Geometry: final body of the model. Coordinates: model frame, mm. Face numbers are marked on the shaded views. Round coordinates to 2 decimals unless told otherwise and drop trailing zeros. Loops run counter-clockwise (first coordinate to the right, second up) from the corner with the lowest first, then second, coordinate; pieces in that order, holes last. Notation, with made-up numbers: (-7, 35) - (-2, 35) arc R28 ccw to (-2, 53) - close; hole circle Ø10 at (-36, -20). An arc over 180 degrees is marked (long way). Answer in a Markdown table with one row per item. Add a question column.
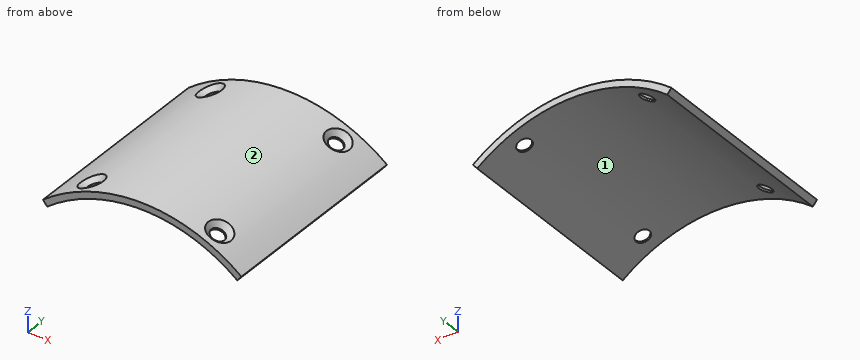
from build123d import *

# Parameters (mm, degrees)
SKETCH1_R           = 76.2
SKETCH1_R_2         = 74.549
BOSS_EXTRUDE1_DEPTH = 254
WRAP2_SECTION_W     = 3.302
WRAP2_SECTION_H     = 101.6
WRAP2_ANGLE         = 76.394372684
SKETCH4_W           = 76.2
SKETCH4_H           = 254


# Read off the part's stored shape, not the designer's step: CSK for 1/4 Flat Head Machine Screw (100)1
with BuildPart() as part:
    # Sketch1 → Boss-Extrude1 (new body)
    with BuildSketch(Plane(origin=(0, 0, 0), x_dir=(1, 0, 0), z_dir=(0, 1, 0))):
        with Locations(Location((0, 0, 0), (0, 0, 270))):
            Circle(SKETCH1_R)
        with Locations(Location((0, 0, 0), (0, 0, 270))):
            Circle(SKETCH1_R_2, mode=Mode.SUBTRACT)
    extrude(amount=BOSS_EXTRUDE1_DEPTH)

    # Wrap2 section (on wrap section) → Wrap2 (revolve)
    with BuildSketch(Plane(origin=(0, 0, 0), x_dir=(0.6183698030697371, 0, 0.7858872607769479), z_dir=(0.7858872607769479, 0, -0.6183698030697371))):
        with Locations((77.851, -127)):
            Rectangle(WRAP2_SECTION_W, WRAP2_SECTION_H)
    revolve(axis=Axis((0, 0, 0), (0, -1, 0)), revolution_arc=WRAP2_ANGLE)

    # Sketch4 → Cut-Revolve1 (revolve, cut)
    with BuildSketch(Plane(origin=(0, 0, 0), x_dir=(0, 0, -1), z_dir=(1, 0, 0))):
        with Locations((38.1, 127)):
            Rectangle(SKETCH4_W, SKETCH4_H)
    revolve(axis=Axis((0, 254, 0), (0, -1, 0)), mode=Mode.SUBTRACT)

    # CSK for 1_4 Flat Head Machine Screw  2 → CSK for 1/4 Flat Head Machine Screw (100)1 (revolve, cut)
    with BuildSketch(Plane(origin=(0, 85.725, 0), x_dir=(0.916971382275524, 0, 0.39895298480863006), z_dir=(0, 1, 0))):
        Polygon((0, -79.50211718), (6.43903965, -79.50211718), (3.57124, -77.095747552), (3.57124, -76.116222895), (0, -76.116222895), align=None)
    revolve(axis=Axis((0, 85.725, 0), (0.3989529848086302, 0, -0.9169713822755242)), mode=Mode.SUBTRACT)

    # CSK for 1_4 Flat Head Machine Screw 3 ou → CSK for 1_4 Flat Head Machine Screw  3 (revolve, cut)
    with BuildSketch(Plane(origin=(0, 85.725, 0), x_dir=(0.9169713822755243, 0, -0.3989529848086292), z_dir=(0, -1, 0))):
        Polygon((6.439064088, 79.502137686), (0, 79.502137686), (0, 76.116222895), (3.57124, 76.116222895), (3.57124, 77.095747552), align=None)
    revolve(axis=Axis((0, 85.725, 0), (0.3989529848086292, 0, 0.9169713822755243)), mode=Mode.SUBTRACT)

    # CSK for 1_4 Flat Head Machine Screw 4 ou → CSK for 1_4 Flat Head Machine Screw  4 (revolve, cut)
    with BuildSketch(Plane(origin=(0, 168.275, 0), x_dir=(0.9169713822755243, 0, -0.3989529848086292), z_dir=(0, -1, 0))):
        Polygon((6.439064088, 79.502137686), (0, 79.502137686), (0, 76.116222895), (3.57124, 76.116222895), (3.57124, 77.095747552), align=None)
    revolve(axis=Axis((0, 168.275, 0), (0.3989529848086292, 0, 0.9169713822755243)), mode=Mode.SUBTRACT)

    # CSK for 1_4 Flat Head Machine Screw 5 ou → CSK for 1_4 Flat Head Machine Screw  5 (revolve, cut)
    with BuildSketch(Plane(origin=(0, 168.275, 0), x_dir=(0.916971382275524, 0, 0.39895298480863006), z_dir=(0, 1, 0))):
        Polygon((0, -79.50211718), (6.43903965, -79.50211718), (3.57124, -77.095747552), (3.57124, -76.116222895), (0, -76.116222895), align=None)
    revolve(axis=Axis((0, 168.275, 0), (0.3989529848086302, 0, -0.9169713822755242)), mode=Mode.SUBTRACT)


solid = part.part
1) Section A-A, the plane z = 64.5. Return the cut outline in (x, y), and give its area (3 significant figures).
2) Section B-B, the plane y = 149.5. Return the cut outline in (x, z), and give its area (3 significant figures).
3) Contact query for flat-ended pins moving along their axis: pin 1 Ø1 at (y, z) = (114.5, 68.5) entering from -X; pin 2 Ø3 at (y, z) = (165.5, 72.5) entering from -X; pin 3 Ø2 at (y, z) = (124.5, 72) entering from +X. Output: stop coordinate, or through.
4) Pull-direction query (X, two-part tool) for the marked faces 1 and 2; classes: pulls with the +X half, pulls with the -X half, needs draft (parallel to the pull), parting line crosses it, or undercut.
5) Section C-C, the plane x = 14. Return the cut outline in (y, z), and give its area (3 significant figures).
6) Material intervals for line 1 along X through (y, z) = (82, 70); line 2 along X through (y, z) = (88, 66.25); line 3 along Z through (x, y) = (44, 102.5), sorted ascending. Write a range as from..to.
Evaluation:
| question | item | result |
|---|---|---|
| 1 | outline | (-46.48, 76.2) - (-40.57, 76.2) - (-40.57, 177.8) - (-46.48, 177.8) - close; (40.57, 76.2) - (46.48, 76.2) - (46.48, 177.8) - (40.57, 177.8) - close |
| 1 | area | 1,200 mm² |
| 2 | outline | (-49.16, 62.48) - (-47.12, 59.88) arc R76.2 cw to (47.12, 59.88) - (49.16, 62.48) arc R79.5 ccw to start |
| 2 | area | 343 mm² |
| 3 | pin 1 | stops at x = -41.19 |
| 3 | pin 2 | stops at x = -29.91 |
| 3 | pin 3 | stops at x = 35.77 |
| 4 | face 1 | undercut |
| 4 | face 2 | parting line crosses it |
| 5 | outline | (76.2, 74.9) - (177.8, 74.9) - (177.8, 78.26) - (76.2, 78.26) - close |
| 5 | area | 341 mm² |
| 6 | line 1 | x = -37.69..-30.11, 30.11..37.69 |
| 6 | line 2 | x = -43.95..-37.65, 37.65..43.95 |
| 6 | line 3 | z = 62.21..66.22 |
